Here's the drawing with two shaded views (mm, measured from the low corner). I have some questions. A direction names the side the tool comes from. Round coordinates to 2 decimals unless told otherwise and drop trailing zeros. Order: outer loops, then holes, each group sorted by start corner. A loop starts at its lowest first (then second) coordinate and runs counter-clockwise, first axis right, second up.
Q1. We'd pull the mould along X, two halves only. Please class the marked faces 1, 2 and 3: pulls with the +X half, pulls with the -X half, needs draft (parallel to the pull), parting line crosses it, or undercut.
Q2. Will these pins go through, and if not, where does the flat tip stop? P1, Ø8, axis at x = 32.5, z = 59, coming from the -Y side; P2, Ø7, axis at y = 16, z = 40.5, coming from the +X side; P3, Ø2, axis at y = 12, z = 10, coming from the +X side (1 decimal); P4, Ø12.5, axis at x = 38.5, y = 7, coming from the -Z side.
Q3. If we section it at B-B (y = 11.5): Please give me the cut outline in (x, z) (1 decimal), plus the area to 3 significant figures.
Q4. If we section it at A-A (y = 3.75): Please give me the cut outline in (x, z) (1 decimal).
Q5. For the marked faces 4 and 5, which set-ups out of +Z, -Z, +X, -X, +Y, -Y let a thin tool reach every point of the face, with its end or its side?
Q6. If I drill on line 1 (Y direction, x = 12, z = 14.5); line 2 (Z direction, x = 14.5, y = 7.5) (1 decimal); line 3 (X direction, y = 11, z = 43.5) (1 decimal), over which ranges is the centre line in solid material (lowest first)?
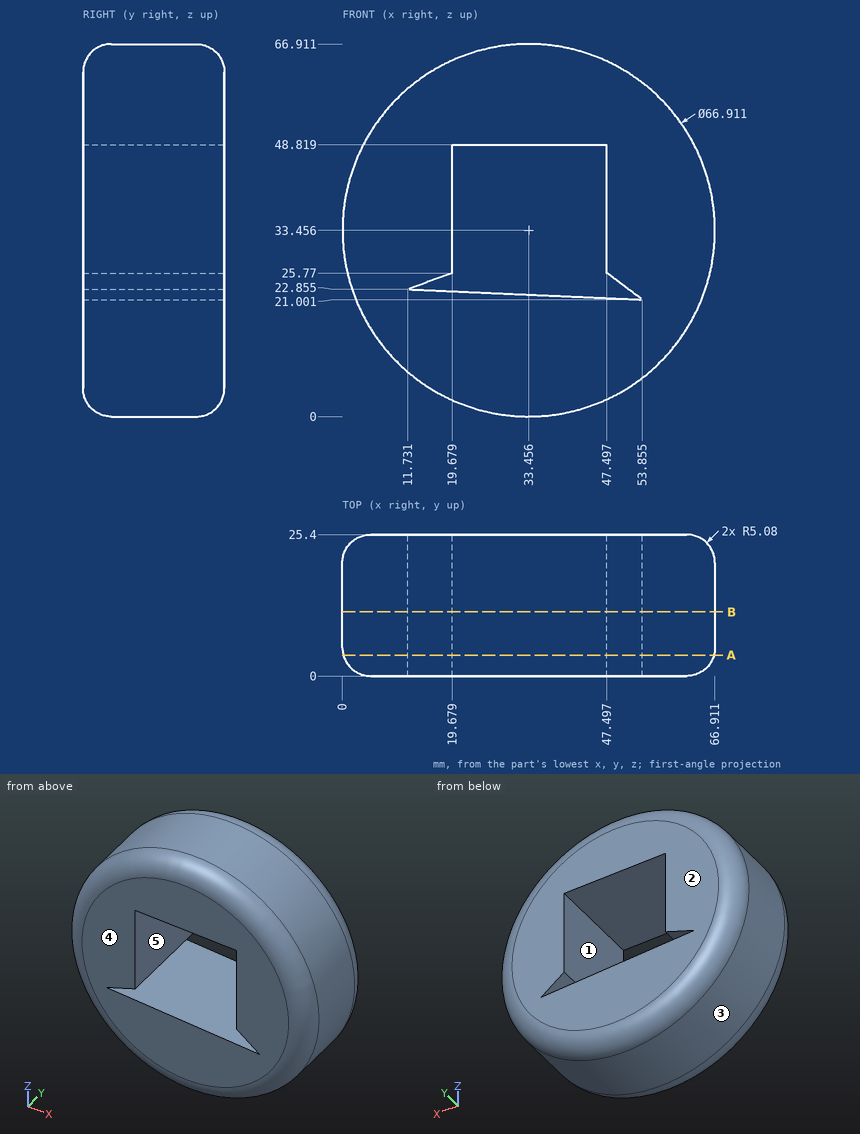
Solution:
1. face 1: undercut
1. face 2: needs draft
1. face 3: parting line crosses it
2. P1: stops at y = 0
2. P2: stops at x = 66.72
2. P3: stops at x = 58.3
2. P4: stops at z = 0
3. outline: circle Ø66.9 at (33.5, 33.5); hole (11.7, 22.9) - (53.9, 21) - (47.5, 25.8) - (47.5, 48.8) - (19.7, 48.8) - (19.7, 25.8) - close
3. area: 2,740 mm2
4. outline: circle Ø66.6 at (33.5, 33.5); hole (11.7, 22.9) - (53.9, 21) - (47.5, 25.8) - (47.5, 48.8) - (19.7, 48.8) - (19.7, 25.8) - close
5. face 4: +Z, -Z, +X, -X, -Y
5. face 5: +Y, -Y
6. line 1: y = 0.01 to 25.39
6. line 2: z = 5.9 to 22.7, 23.9 to 61
6. line 3: x = 1.5 to 19.7, 47.5 to 65.4
